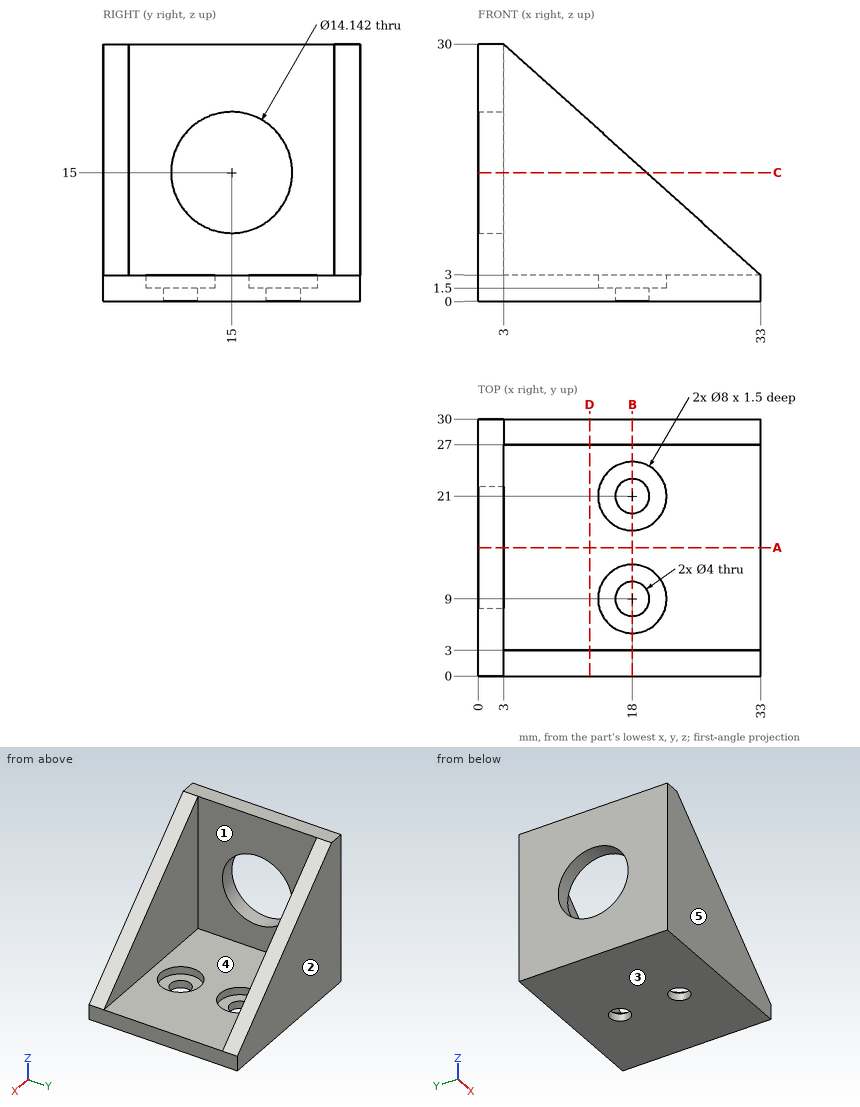
Source: three-view drawing plus pictorial views. Frame: mm from the lowest corner of the part. A direction names the side the tool comes from. Coordinates: 2 decimals unless noted, no trailing zeros. Loops run counter-clockwise (first coordinate to the right, second up) from the corner with the lowest first, then second, coordinate; pieces in that order, holes last. Notation, with made-up numbers: (-26, 30) -> (-10, 30) arc R17 ccw to (-10, 59) -> close; hole circle Ø2 at (-27, 6). An arc over 180 degrees is marked (long way). Answer in a Markdown table with one row per item. Add a question column.
Q1. Section B-B on x = 18. Return the cut outline in (y, z).
Q2. Section A-A on y = 15. Return the cut outline in (x, z).
Q3. Ray query, line 1 along Y through (x, z) = (18, 2.2); line 2 along Y through (x, z) = (18, 0.55); line 3 along Y through (x, z) = (20, 9.5). Return the intervals inside material, ascending.
Q4. Pull-direction query (Y, two-part tool) for the marked faces 1, 2 and 3; classes: pulls with the +Y half, pulls with the -Y half, needs draft (parallel to the pull), parting line crosses it, or undercut.
Q5. Reachability of the marked faces 4 and 5 from +Z, -Z, +X, -X, +Y, -Y: full face, straight path, thin tool, end or side. Return the list, or none.
Q6. Section C-C on z = 15. Return the cut outline in (x, y).
Q7. Section D-D on x = 13. Return the cut outline in (y, z), and give its area (3 significant figures).
Q8. Contact query for flat-ended pins moving along their axis: pin 1 Ø6 at (x, y) = (13, 16) entering from -Z; pin 2 Ø1.5 at (y, z) = (8, 12.5) entering from +X; pin 3 Ø10 at (x, y) = (10, 11) entering from +Z. Output: stop coordinate, or through.
Computed values:
| question | item | result |
|---|---|---|
| 1 | outline | (0, 0) -> (7, 0) -> (7, 1.5) -> (5, 1.5) -> (5, 3) -> (3, 3) -> (3, 16.5) -> (0, 16.5) -> close; (11, 0) -> (19, 0) -> (19, 1.5) -> (17, 1.5) -> (17, 3) -> (13, 3) -> (13, 1.5) -> (11, 1.5) -> close; (23, 0) -> (30, 0) -> (30, 16.5) -> (27, 16.5) -> (27, 3) -> (25, 3) -> (25, 1.5) -> (23, 1.5) -> close |
| 2 | outline | (0, 0) -> (33, 0) -> (33, 3) -> (3, 3) -> (3, 7.93) -> (0, 7.93) -> close; (0, 22.07) -> (3, 22.07) -> (3, 30) -> (0, 30) -> close |
| 3 | line 1 | y = 0 to 5, 13 to 17, 25 to 30 |
| 3 | line 2 | y = 0 to 7, 11 to 19, 23 to 30 |
| 3 | line 3 | y = 0 to 3, 27 to 30 |
| 4 | face 1 | undercut |
| 4 | face 2 | pulls with the +Y half |
| 4 | face 3 | needs draft |
| 5 | face 4 | +Z, +X |
| 5 | face 5 | +Z, -Z, +X, -X, -Y |
| 6 | outline | (0, 0) -> (19.67, 0) -> (19.67, 3) -> (3, 3) -> (3, 7.93) -> (0, 7.93) -> close; (0, 22.07) -> (3, 22.07) -> (3, 27) -> (19.67, 27) -> (19.67, 30) -> (0, 30) -> close |
| 7 | outline | (0, 0) -> (30, 0) -> (30, 21) -> (27, 21) -> (27, 3) -> (3, 3) -> (3, 21) -> (0, 21) -> close |
| 7 | area | 198 mm^2 |
| 8 | pin 1 | stops at z = 0 |
| 8 | pin 2 | stops at x = 3 |
| 8 | pin 3 | stops at z = 3 |
